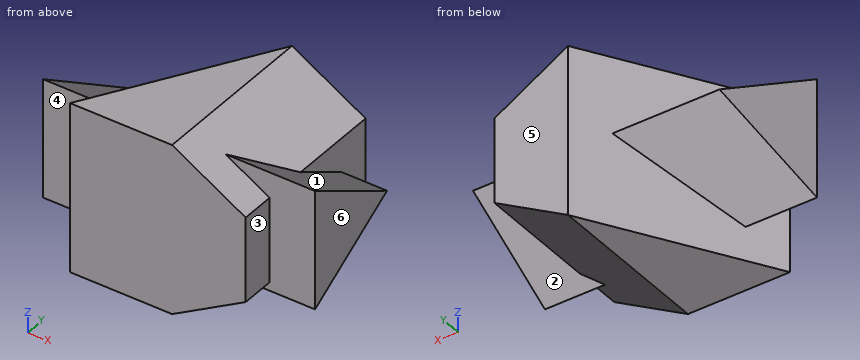
from build123d import *

# Parameters (mm, degrees)
EXTRUDE1_DEPTH = 100
EXTRUDE2_DEPTH = 101
EXTRUDE3_START = -30
EXTRUDE3_DEPTH = 160
EXTRUDE4_DEPTH = 160


with BuildPart() as part:
    # Sketch1 → Extrude1 (new body)
    with BuildSketch(Plane(origin=(0, 0, 0), x_dir=(1, 0, 0), z_dir=(0, 1, 0))):
        Polygon((60, 0), (103.301270189, 25), (103.301270189, 75), (60, 100), (0, 100), (0, 0), align=None)
    extrude(amount=EXTRUDE1_DEPTH)

    # Sketch2 → Extrude2 (cut, through all)
    with BuildSketch(Plane.XY):
        Polygon((60, 100), (0, 0), (0, 100), align=None)
    extrude(amount=-EXTRUDE2_DEPTH, mode=Mode.SUBTRACT)

    # Sketch3 → Extrude3 (add)
    with BuildSketch(Plane(origin=(0, 0, 0), x_dir=(0, 0, -1), z_dir=(1, 0, 0)).offset(EXTRUDE3_START)):
        Polygon((45, 80), (80, 20), (10, 20), align=None)
    extrude(amount=EXTRUDE3_DEPTH)

    # Sketch4 → Extrude4 (cut)
    with BuildSketch(Plane.XY):
        Polygon((-30, 20), (-15, 80), (-30, 80), align=None)
    extrude(amount=-EXTRUDE4_DEPTH, mode=Mode.SUBTRACT)


solid = part.part
Input: part model. Units: mm. Frame: model coordinates. Face numbers are marked on the shaded views. A direction names the side the tool comes from. Coordinates: 2 decimals unless noted, no trailing zeros. Loops run counter-clockwise (first coordinate to the right, second up) from the corner with the lowest first, then second, coordinate; pieces in that order, holes last. Notation, with made-up numbers: (36.5, -24.5) -> (63.5, -24.5) arc R26 ccw to (63.5, -3.5) -> close; hole circle Ø7 at (-37.75, 82.25). An arc over 180 degrees is marked (long way). One line per item, written item: value.
(1) Cut plane B-B (x = 26). Output: boundary loops of the cut face in (y, z), then the cut area to 3 significant figures.
Answer below:
outline: (0, -100) -> (43.33, -100) -> (43.33, -66.39) -> (80, -45) -> (43.33, -23.61) -> (43.33, 0) -> (0, 0) -> close
area: 5,120 mm2
(2) Pin query (flat end, axial travel): pin 1 Ø5 at (y, z) = (45, -13.5) entering from +X; pin 2 Ø2 at (x, y) = (88.5, 55) entering from +Z; pin 3 Ø8 at (x, y) = (104.5, 59) entering from +Z. Return the tip coordinate at first contact, or that it passes through.
Answer below:
pin 1: stops at x = 87.71
pin 2: stops at z = -15.88
pin 3: stops at z = -23.38
(3) Set-up query: the marked faces 1, 2 and 3. Return all of +Z, -Z, +X, -X, +Y, -Y with unobstructed straight access to the full face (end or side cutting, diameter ignored); none if empty.
Answer below:
face 1: +Z, +X, +Y
face 2: -Z, +X, +Y
face 3: +Z, -Z, +X, -Y
(4) Cut plane C-C (y = 6). Output: boundary loops of the cut face in (x, z).
Answer below:
outline: (3.6, -100) -> (60, -100) -> (103.3, -75) -> (103.3, -25) -> (60, 0) -> (3.6, 0) -> close
(5) Draft query along Y for the marked faces 4, 5 and 6. Return one class per face: pulls with the +Y half, pulls with the -Y half, needs draft (parallel to the pull), parting line crosses it, or undercut.
Answer below:
face 4: undercut
face 5: pulls with the +Y half
face 6: needs draft
(6) Cut plane A-A (z = -66). Output: boundary loops of the cut face in (x, y).
Answer below:
outline: (-30, 20) -> (12, 20) -> (0, 0) -> (103.3, 0) -> (103.3, 20) -> (130, 20) -> (130, 44) -> (103.3, 44) -> (103.3, 100) -> (60, 100) -> (26.4, 44) -> (-24, 44) -> close
(7) Cut plane D-D (x = 51). Output: boundary loops of the cut face in (y, z).
Answer below:
outline: (0, -100) -> (85, -100) -> (85, 0) -> (0, 0) -> close
(8) Ray query, line 1 along Z through (x, y) = (13.5, 79.5); line 2 along X through (y, z) = (19, -18.5); line 3 along X through (y, z) = (14.5, -29.5). Return the intervals inside material, ascending.
Answer below:
line 1: z = -45.29 to -44.71
line 2: x = 11.4 to 92.04
line 3: x = 8.7 to 103.3
